```python
from build123d import *

# Parameters (mm, degrees)
EXTRUDE_1_DEPTH          = 20
SKETCH_2_R               = 3
SKETCH_2_R_2             = 1.75
CUT_EXTRUDE_1_DEPTH      = 112
CUT_EXTRUDE_2_DEPTH      = 123
CUT_EXTRUDE_2_DEPTH_BACK = 61
SKETCH_5_W               = 18
SKETCH_5_H               = 40
EXTRUDE_3_DEPTH          = 15
CUT_EXTRUDE_3_DEPTH      = 141.356688476
CUT_EXTRUDE_3_DEPTH_BACK = 141.356688476
SKETCH_6_R               = 2
CUT_EXTRUDE_4_DEPTH      = 141.356688476
CUT_EXTRUDE_4_DEPTH_BACK = 141.356688476
FILLET_1_R               = 6
FILLET_2_R               = 12
SKETCH_9_R               = 7.5
CUT_EXTRUDE_6_DEPTH      = 8
SKETCH_10_R              = 3
CUT_EXTRUDE_7_DEPTH      = 16
SKETCH_11_R              = 1.75
SKETCH_11_R_2            = 3
CUT_EXTRUDE_8_DEPTH      = 23
SKETCH_12_R              = 3.5
CUT_EXTRUDE_9_DEPTH      = 16
SKETCH_14_R              = 3.5
CUT_EXTRUDE_10_DEPTH     = 45


with BuildPart() as part:
    # 草图1 → 凸台-拉伸1 (new, symmetric)
    with BuildSketch(Plane(origin=(0, 0, 0), x_dir=(1, 0, 0), z_dir=(0, 1, 0))):
        Polygon((-18, 0), (0, 0), (0, 90), (-100, 90), (-100, 0), (-82, 0), (-82, 72), (-18, 72), align=None)
    extrude(amount=EXTRUDE_1_DEPTH, both=True)

    # 草图2 → 切除-拉伸1 (cut)
    with BuildSketch(Plane.ZY.offset(100)):
        with Locations((-7, 0)):
            Circle(SKETCH_2_R)
        with Locations((-7, 15.5)):
            Circle(SKETCH_2_R_2)
        with Locations((-7, -15.5)):
            Circle(SKETCH_2_R_2)
    extrude(amount=-CUT_EXTRUDE_1_DEPTH, mode=Mode.SUBTRACT)

    # 草图4 → 切除-拉伸2 (cut, two sides: drawn at the far end of the back side and taken through both)
    with BuildSketch(Plane.ZY.offset(18).offset(-CUT_EXTRUDE_2_DEPTH_BACK)):
        with BuildLine():
            Line((-62, 12.5), (-33, 12.5))
            ThreePointArc((-33, 12.5), (-30.878679656, 11.621320344), (-30, 9.5))
            Line((-30, 9.5), (-30, -9.5))
            ThreePointArc((-30, -9.5), (-30.878679656, -11.621320344), (-33, -12.5))
            Line((-33, -12.5), (-62, -12.5))
            ThreePointArc((-62, -12.5), (-64.121320344, -11.621320344), (-65, -9.5))
            Line((-65, -9.5), (-65, 9.5))
            ThreePointArc((-65, 9.5), (-64.121320344, 11.621320344), (-62, 12.5))
        make_face()
    extrude(amount=CUT_EXTRUDE_2_DEPTH + CUT_EXTRUDE_2_DEPTH_BACK, mode=Mode.SUBTRACT)

    # 草图5 → 凸台-拉伸3 (add)
    with BuildSketch(Plane.XY):
        with Locations((-9, 0)):
            Rectangle(SKETCH_5_W, SKETCH_5_H)
        with Locations((-91, 0)):
            Rectangle(SKETCH_5_W, SKETCH_5_H)
    extrude(amount=EXTRUDE_3_DEPTH)

    # 草图6 → 切除-拉伸3 (cut, two sides: drawn at the far end of the back side and taken through both)
    with BuildSketch(Plane(origin=(0, 20, 0), x_dir=(1, 0, 0), z_dir=(0, 1, 0)).offset(-CUT_EXTRUDE_3_DEPTH_BACK)):
        with Locations(Location((-91, 60, 0), (0, 0, 270))):
            Circle(SKETCH_6_R)
        with Locations(Location((-91, 52, 0), (0, 0, 270))):
            Circle(SKETCH_6_R)
        with Locations(Location((-91, 44, 0), (0, 0, 270))):
            Circle(SKETCH_6_R)
        with Locations(Location((-91, 36, 0), (0, 0, 270))):
            Circle(SKETCH_6_R)
        with Locations(Location((-9, 36, 0), (0, 0, 270))):
            Circle(SKETCH_6_R)
        with Locations(Location((-9, 44, 0), (0, 0, 270))):
            Circle(SKETCH_6_R)
        with Locations(Location((-9, 52, 0), (0, 0, 270))):
            Circle(SKETCH_6_R)
        with Locations(Location((-9, 60, 0), (0, 0, 90))):
            Circle(SKETCH_6_R)
    extrude(amount=CUT_EXTRUDE_3_DEPTH + CUT_EXTRUDE_3_DEPTH_BACK, mode=Mode.SUBTRACT)

    # 草图7 → 切除-拉伸4 (cut, two sides: drawn at the far end of the back side and taken through both)
    with BuildSketch(Plane(origin=(0, 20, 0), x_dir=(1, 0, 0), z_dir=(0, 1, 0)).offset(-CUT_EXTRUDE_4_DEPTH_BACK)):
        with BuildLine():
            Line((-90.5, 85.5), (-63.5, 85.5))
            ThreePointArc((-63.5, 85.5), (-59, 81), (-63.5, 76.5))
            Line((-63.5, 76.5), (-90.5, 76.5))
            ThreePointArc((-90.5, 76.5), (-95, 81), (-90.5, 85.5))
        make_face()
        with BuildLine():
            Line((-9.5, 85.5), (-36.5, 85.5))
            ThreePointArc((-36.5, 85.5), (-41, 81), (-36.5, 76.5))
            Line((-36.5, 76.5), (-9.5, 76.5))
            ThreePointArc((-9.5, 76.5), (-5, 81), (-9.5, 85.5))
        make_face()
    extrude(amount=CUT_EXTRUDE_4_DEPTH + CUT_EXTRUDE_4_DEPTH_BACK, mode=Mode.SUBTRACT)

    # 圆角1
    fillet_1_edges = [part.edges().sort_by_distance(p)[0] for p in [
        (-18, 0, -72),
        (-82, 0, -72),
        (-100, 0, -90),
        (0, 0, -90),
    ]]
    fillet(fillet_1_edges, radius=FILLET_1_R)

    # 圆角2
    fillet_2_edges = [part.edges().sort_by_distance(p)[0] for p in [
        (-9, -20, 15),
        (-9, 20, 15),
        (-91, -20, 15),
        (-91, 20, 15),
    ]]
    fillet(fillet_2_edges, radius=FILLET_2_R)

    # 草图9 → 切除-拉伸6 (cut)
    with BuildSketch(Plane(origin=(0, 0, -90), x_dir=(-1, 0, 0), z_dir=(0, 0, -1))):
        with Locations((50, 0)):
            Circle(SKETCH_9_R)
    extrude(amount=-CUT_EXTRUDE_6_DEPTH, mode=Mode.SUBTRACT)

    # 草图10 → 切除-拉伸7 (cut)
    with BuildSketch(Plane.XY.offset(-72)):
        with Locations((-50, 0)):
            Circle(SKETCH_10_R)
    extrude(amount=-CUT_EXTRUDE_7_DEPTH, mode=Mode.SUBTRACT)

    # 草图11 → 切除-拉伸8 (cut)
    with BuildSketch(Plane.XY.offset(-72)):
        with Locations((-34.5, 0)):
            Circle(SKETCH_11_R)
        with Locations((-65.5, 0)):
            Circle(SKETCH_11_R)
        with Locations((-50, 0)):
            Circle(SKETCH_11_R_2)
    extrude(amount=-CUT_EXTRUDE_8_DEPTH, mode=Mode.SUBTRACT)

    # 草图12 → 切除-拉伸9 (cut)
    with BuildSketch(Plane(origin=(0, 0, -90), x_dir=(-1, 0, 0), z_dir=(0, 0, -1))):
        with Locations((34.5, 0)):
            Circle(SKETCH_12_R)
        with Locations((65.5, 0)):
            Circle(SKETCH_12_R)
    extrude(amount=-CUT_EXTRUDE_9_DEPTH, mode=Mode.SUBTRACT)

    # 草图14 → 切除-拉伸10 (cut, symmetric)
    with BuildSketch(Plane(origin=(-50, 0, 0), x_dir=(0, 0, -1), z_dir=(1, 0, 0))):
        with Locations((7, 15.5)):
            Circle(SKETCH_14_R)
        with Locations((7, -15.5)):
            Circle(SKETCH_14_R)
    extrude(amount=CUT_EXTRUDE_10_DEPTH, both=True, mode=Mode.SUBTRACT)


solid = part.part
```
For this review, take the finished solid that the model builds, in its own axes (mm). A direction names the side the tool comes from. Coordinates: 2 decimals unless noted, no trailing zeros. Order: outer loops, then holes, each group sorted by start corner. A loop starts at its lowest first (then second) coordinate and runs counter-clockwise, first axis right, second up. Notation, with made-up numbers: (15.25, 46.25) -> (57.25, 46.25) arc R24 cw to (57.25, 81.25) -> close; hole circle Ø9 at (77, 15). An arc over 180 degrees is marked (long way). Use CSV: the item, a comma, the result in double quotes. Start each with the question number.
Item 1: Wall thickness on probe 1 along X at (y, z) = (-14, -44); probe 2 along X at (y, z) = (-16.5, -64.5); probe 3 along Y at (x, z) = (-89, -7): over which ranges is each line inside the solid? List them lowest first.
Item 2: We need section C-C, the plane z = 8.5. Give the boundary of the cut face in (x, y).
Item 3: We need section B-B, the plane x = -51.5. Give the boundary of the cut face in (y, z), then the cut area to 3 significant figures.
Item 4: We need section A-A, the plane z = -36. Give the number of separate pieces and of enclosed holes in the cut face, then the cut area to 3 significant figures.
Item 5: Draft analysis for pull direction Y (two halves, no side actions). For faces 4 (the face through (-9, -12.5, -47)), 5 (the face through (-7.648, -16.302, -53.474)), 6 (the face through (-90.87, -16.58, 11.39)), 7 (the face through (-8.87, 16.58, 11.39)), state which applies: pulls with the +Y half, pulls with the -Y half, needs draft (parallel to the pull), parting line crosses it, or undercut.
Item 6: Insertion check: pin 1 (8 mm diameter, centred on y = -3.5, z = -20.5, fed in from +X); pin 2 (1.5 mm diameter, centred on x = -80.5, z = -51, fed in from -Y); pin 3 (10 mm diameter, centred on x = -49, y = 7, fed in from +Z). Each pin has a flat end and moves straight along its axis. Give the tip position at first contact, or say it passes through.
Item 7: For faces 1 (the face through (-88, 19, -7)), 2 (the face through (-89, 16, -60)), 3 (the face through (-8.87, 11.64, -30.9)), list the 3-axis set-ups (+Z, -Z, +X, -X, +Y, -Y) from which the entire face can be reached by the end or side of a thin tool; tool diameter is ignored.
Derived:
1,probe 1,"x = -100 to -93, -89 to -82, -18 to -11, -7 to 0"
1,probe 2,"x = -100 to -82, -18 to 0"
1,probe 3,"y = -20 to -19, -12 to -3, 3 to 12, 19 to 20"
2,outline,"(-100, -18.67) -> (-82, -18.67) -> (-82, 18.67) -> (-100, 18.67) -> close; (-18, -18.67) -> (0, -18.67) -> (0, 18.67) -> (-18, 18.67) -> close"
3,outline,"(-20, -90) -> (-7.35, -90) -> (-7.35, -82) -> (-2.6, -82) -> (-2.6, -72) -> (-20, -72) -> close; (2.6, -82) -> (7.35, -82) -> (7.35, -90) -> (20, -90) -> (20, -72) -> (2.6, -72) -> close"
3,area,"550 mm^2"
4,separate pieces,"8"
4,enclosed holes,"0"
4,area,"420 mm^2"
5,face 4,"undercut"
5,face 5,"needs draft"
5,face 6,"pulls with the -Y half"
5,face 7,"pulls with the +Y half"
6,pin 1,"stops at x = 0"
6,pin 2,"passes through"
6,pin 3,"stops at z = -72"
7,face 1,"none"
7,face 2,"+Y, -Y"
7,face 3,"+X, -X"
